CAD build for the part. Positions are in the model's coordinates, mm. Face numbers are marked on the shaded views. A direction names the side the tool comes from. Give positions to 0.01 mm unless a question says otherwise; leave off trailing zeros. Loops run counter-clockwise (first coordinate to the right, second up) from the corner with the lowest first, then second, coordinate; pieces in that order, holes last.
```python
from build123d import *

# Parameters (mm, degrees)
SKETCH2_R          = 6.5
CUT_EXTRUDE1_DEPTH = 254


with BuildPart() as part:
    # Sketch1 → Revolve1 (revolve)
    with BuildSketch(Plane.XY):
        Polygon((-182.5, 10), (-182.5, 38), (-96.5, 38), (-96.5, 65), (33.5, 65), (33.5, 105), (70.5, 105), (70.5, 33), (130.5, 33), (130.5, 18), (182.5, 18), (182.5, 10), align=None)
    revolve(axis=Axis((-194.069566155, 0, 0), (1, 0, 0)))

    # Sketch2 → Cut-Extrude1 (cut, through all)
    with BuildSketch(Plane(origin=(70.5, 0, 0), x_dir=(0, 0, -1), z_dir=(1, 0, 0))):
        with Locations((0, 80)):
            Circle(SKETCH2_R)
        with Locations((56.568542495, 56.568542495)):
            Circle(SKETCH2_R)
        with Locations((80, 0)):
            Circle(SKETCH2_R)
        with Locations((56.568542495, -56.568542495)):
            Circle(SKETCH2_R)
        with Locations((0, -80)):
            Circle(SKETCH2_R)
        with Locations((-56.568542495, -56.568542495)):
            Circle(SKETCH2_R)
        with Locations((-80, 0)):
            Circle(SKETCH2_R)
        with Locations((-56.568542495, 56.568542495)):
            Circle(SKETCH2_R)
    extrude(amount=-CUT_EXTRUDE1_DEPTH, mode=Mode.SUBTRACT)


solid = part.part
```
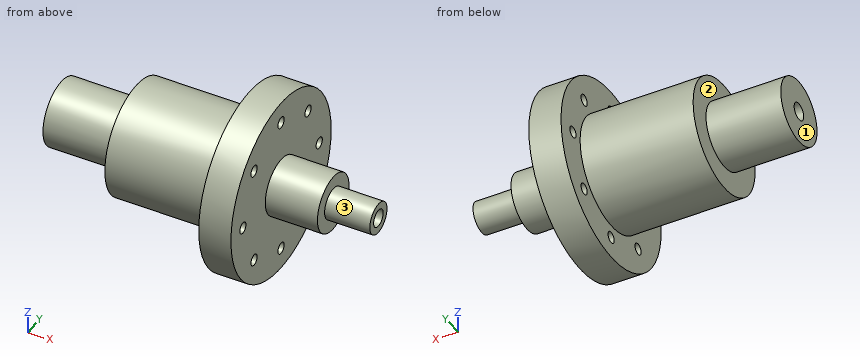
1. Drop flat-ended pins along their axis: pin 1 (8 mm diameter, centred on y = -75.5, z = 66.5, fed in from +X); pin 2 (11.5 mm diameter, centred on y = 56.57, z = -56.57, fed in from -X); pin 3 (8 mm diameter, centred on x = 7, y = -41.5, fed in from -Z); pin 4 (15 mm diameter, centred on y = 80, z = 0, fed in from -X). Give the stop position or say it passes through.
Responses:
pin 1: stops at x = 70.5
pin 2: passes through
pin 3: stops at z = -53.09
pin 4: stops at x = 33.5
2. Saw through at D-D, the plane z = 81. List the corners of the cut face in (x, y), and give its area (3 significant figures).
Responses:
outline: (33.5, -66.81) - (70.5, -66.81) - (70.5, -6.42) - (33.5, -6.42) - close; (33.5, 6.42) - (70.5, 6.42) - (70.5, 66.81) - (33.5, 66.81) - close
area: 4,470 mm2
3. Probe line 1 along Z through (x, y) = (60.5, -2); line 2 along Z through (x, y) = (-97, 0); line 3 along X through (y, z) = (-46, 55). List the from-to ranges inside material, lowest first.
Responses:
line 1: z = -104.98 to -86.18, -73.82 to -9.8, 9.8 to 73.82, 86.18 to 104.98
line 2: z = -38 to -10, 10 to 38
line 3: x = 33.5 to 70.5
4. Saw through at A-A, the plane y = 0. Count the separate pieces of the cut face and the enclosed holes in it, and give its area (3 significant figures).
Responses:
separate pieces: 4
enclosed holes: 0
area: 28,800 mm2
5. Tool access for the marked faces 1, 2 and 3: list every direction of +Z, -Z, +X, -X, +Y, -Y with a clear straight run to the whole face (end or side of a thin tool).
Responses:
face 1: +Z, -Z, -X, +Y, -Y
face 2: -X
face 3: +X
